Could you check a few things on this model? Use its own coordinates, in mm. Face numbers are marked on the shaded views. Give positions to 0.01 mm unless a question says otherwise; leave off trailing zeros. Order: outer loops, then holes, each group sorted by start corner. A loop starts at its lowest first (then second) coordinate and runs counter-clockwise, first axis right, second up. Notation, with made-up numbers: (-12, 82) - (40, 82) arc R18 cw to (40, 117) - close; hole circle Ø5 at (23.25, 64). An arc over 180 degrees is marked (long way). Put each result on its own line as item: value.
Autodesk Inventor part; units mm, degrees
ref_plane "YZ Plane" through (0, 0, 0) normal (1, 0, 0) x (0, 1, 0)
ref_plane "XZ Plane" through (0, 0, 0) normal (0, 1, 0) x (-1, 0, 0)
ref_plane "XY Plane" through (0, 0, 0) normal (0, 0, 1) x (1, 0, 0)
sketch "Sketch1" plane through (0, 0, 0) normal (0, 0, 1) x (1, 0, 0)
  line L0 (0, 0) -> (0, 101.6)
  line L1 (0, 101.6) -> (25.4, 101.6)
  line L2 (25.4, 101.6) -> (25.4, 65.5898)
  line L3 (50.8, 65.5898) -> (50.8, 78.2898)
  line L4 (60.96, 78.2898) -> (60.96, 65.5898)
  line L5 (25.0337, 0) -> (0, 0)
  arc A0 (38.1, 52.8898) -> (50.8, 65.5898) centre (38.1, 65.5898) ccw
  arc A1 (25.4, 65.5898) -> (38.7011, 52.904) centre (38.1, 65.5898) ccw
  arc A2 (60.96, 78.2898) -> (50.8, 78.2898) centre (55.88, 78.2898) ccw
  line L6 (25.4, 65.5898) -> (50.8, 65.5898) construction
  arc A3 (35.4242, 23.2943) -> (60.96, 65.5898) centre (13.1646, 65.5898) ccw
  arc A4 (35.4242, 23.2943) -> (25.0337, 6.0842) centre (44.4817, 6.0842) ccw
  line L7 (25.0337, 6.0842) -> (25.0337, 0)
  dimension "d0" = 101.6
  dimension "d2" = 25.4
  dimension "d4" = 25.4
  dimension "d6" = 10.16
  dimension "d9" = 12.7
  dimension "d10" = 12.7
  dimension "d13" = 60.96
extrude "Extrusion1" add sketch "Sketch1" along normal blind 6.35
properties part number "Can Hook"
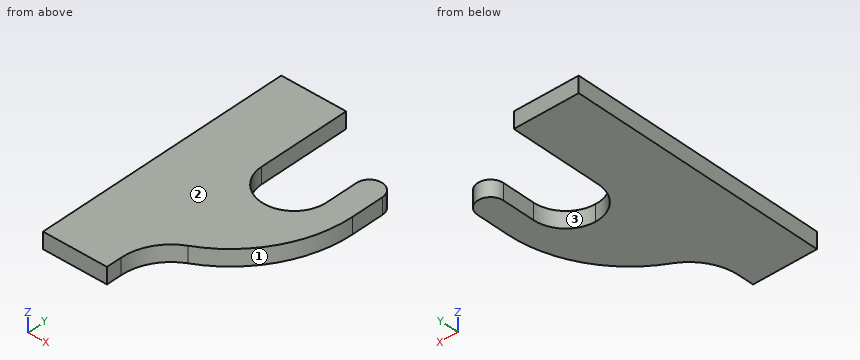
1) I'm going to push a flat-ended pin straight in: pin 1 (6 mm diameter, centred on x = 27.5, y = 90.5, fed in from -Z). Where does the tip first touch, or does it pass through?
Filled in:
pin 1: stops at z = 0
2) If I drill on line 1 (X direction, y = 73, z = 2.75); line 2 (X direction, y = 39, z = 3.75); line 3 (X direction, y = 63.5, z = 2), over which ranges is the centre line in solid material (lowest first)? Write a range as [from, to].
Filled in:
line 1: x = [0, 25.4], [50.8, 60.96]
line 2: x = [0, 52.88]
line 3: x = [0, 25.57], [50.63, 60.91]
3) Suppose I cut it at D-D, the plane x = 30. List the corners of the cut face in (y, z) for me.
Filled in:
outline: (19.07, 0) - (55.81, 0) - (55.81, 6.35) - (19.07, 6.35) - close
4) We'd pull the mould along X, two halves only. Please class the marked faces 1, 2 and 3: pulls with the +X half, pulls with the -X half, needs draft (parallel to the pull), parting line crosses it, or undercut.
Filled in:
face 1: pulls with the +X half
face 2: needs draft
face 3: undercut
5) Suppose I cut it at A-A, the plane z = 3.5. List the corners of the cut face in (x, y) for me, and give its area (3 significant figures).
Filled in:
outline: (0, 0) - (25.03, 0) - (25.03, 6.08) arc R19.45 cw to (35.42, 23.29) arc R47.8 ccw to (60.96, 65.59) - (60.96, 78.29) arc R5.08 ccw to (50.8, 78.29) - (50.8, 65.59) arc R12.7 cw to (38.1, 52.89) arc R12.7 cw to (25.4, 65.59) - (25.4, 101.6) - (0, 101.6) - close
area: 3,730 mm^2
6) Suppose I cut it at C-C, the plane y = 28.5. List the corners of the cut face in (x, z) for me.
Filled in:
outline: (0, 0) - (43.31, 0) - (43.31, 6.35) - (0, 6.35) - close
7) Suppose I cut it at B-B, the plane y = 57. List the corners of the cut face in (x, z) for me, and give its area (3 significant figures).
Filled in:
outline: (0, 0) - (28.75, 0) - (28.75, 6.35) - (0, 6.35) - close; (47.45, 0) - (60.18, 0) - (60.18, 6.35) - (47.45, 6.35) - close
area: 263 mm^2
